from build123d import *

# Parameters (mm, degrees)
F0_R     = 6.35
F1_DEPTH = 19.05


with BuildPart() as f1:
    # F0 (on Front) → F1 (new body)
    with BuildSketch(Plane.XZ):
        with BuildLine():
            ThreePointArc((6.35, -50.8), (4.490128, -46.309872), (0, -44.45))
            ThreePointArc((0, -44.45), (-4.490128, -55.290128), (6.35, -50.8))
        make_face()
        with Locations((-50.8, 0)):
            Circle(F0_R)
        with BuildLine():
            ThreePointArc((6.35, 50.8), (-4.490128, 55.290128), (0, 44.45))
            ThreePointArc((0, 44.45), (4.490128, 46.309872), (6.35, 50.8))
        make_face()
        with BuildLine():
            ThreePointArc((57.15, 0), (50.8, 6.35), (44.45, 0))
            ThreePointArc((44.45, 0), (50.8, -6.35), (57.15, 0))
        make_face()
        with BuildLine():
            ThreePointArc((12.883376, 50.8), (9.109922, 59.909922), (0, 63.683376))
            ThreePointArc((0, 63.683376), (-9.109922, 59.909922), (-12.883376, 50.8))
            ThreePointArc((-12.883376, 50.8), (-21.70632, 21.661631), (-50.8, 12.692425))
            ThreePointArc((-50.8, 12.692425), (-59.7749, 8.9749), (-63.492425, 0))
            ThreePointArc((-63.492425, 0), (-59.7749, -8.9749), (-50.8, -12.692425))
            ThreePointArc((-50.8, -12.692425), (-22.664281, -22.614792), (-12.883376, -50.8))
            ThreePointArc((-12.883376, -50.8), (-9.109922, -59.909922), (0, -63.683376))
            ThreePointArc((0, -63.683376), (9.109922, -59.909922), (12.883376, -50.8))
            ThreePointArc((12.883376, -50.8), (22.285467, -22.332575), (50.8, -13.074334))
            ThreePointArc((50.8, -13.074334), (60.04495, -9.24495), (63.874334, 0))
            ThreePointArc((63.874334, 0), (60.04495, 9.24495), (50.8, 13.074334))
            ThreePointArc((50.8, 13.074334), (21.896637, 21.941776), (12.883376, 50.8))
        make_face()
        with BuildLine():
            ThreePointArc((6.35, -50.8), (-4.490128, -55.290128), (0, -44.45))
            ThreePointArc((0, -44.45), (4.490128, -46.309872), (6.35, -50.8))
        make_face(mode=Mode.SUBTRACT)
        with Locations((-50.8, 0)):
            Circle(F0_R, mode=Mode.SUBTRACT)
        with BuildLine():
            ThreePointArc((0, 12.7), (8.980256, 8.980256), (12.7, 0))
            ThreePointArc((12.7, 0), (8.980256, -8.980256), (0, -12.7))
            ThreePointArc((0, -12.7), (-8.980256, -8.980256), (-12.7, 0))
            ThreePointArc((-12.7, 0), (-8.980256, 8.980256), (0, 12.7))
        make_face(mode=Mode.SUBTRACT)
        with BuildLine():
            ThreePointArc((6.35, 50.8), (4.490128, 46.309872), (0, 44.45))
            ThreePointArc((0, 44.45), (-4.490128, 55.290128), (6.35, 50.8))
        make_face(mode=Mode.SUBTRACT)
        with BuildLine():
            ThreePointArc((57.15, 0), (50.8, -6.35), (44.45, 0))
            ThreePointArc((44.45, 0), (50.8, 6.35), (57.15, 0))
        make_face(mode=Mode.SUBTRACT)
    extrude(amount=F1_DEPTH)


solid = f1.part
Design review of the part built by this model. Coordinates are the model's own, in mm. Round coordinates to 2 decimals unless told otherwise and drop trailing zeros. Write each loop counter-clockwise with the first axis right and the second up, starting at its lowest first coordinate (ties: lowest second). Pieces come first, ordered by that corner, then holes. Notation, with made-up numbers: (61, 6) - (111, 6) arc R3 ccw to (111, 10) - close; hole circle Ø6 at (18.5, 4). An arc over 180 degrees is marked (long way). Return JSON: item names as keys, results as strings. Group by question number.
Item 1: We need section A-A on y = -7.25. Write out the cut boundary in (x, z), and give its area (3 significant figures).
Item 2: We need section B-B on x = 20.5. Write out the cut boundary in (y, z).
Item 3: For probe 1 along Z at (x, y) = (2, -16); probe 2 along Z at (x, y) = (50.8, -10); probe 3 along Z at (x, y) = (-50.8, -4.5), list the stretches that pass through material, from the lowest coordinate up. Write a range as [from, to].
Item 4: The part is to be moulded in two halves that separate along Z. For faces 1 (the face through (-21.396, -9.392, 21.978)), 2 (the face through (-14, -19.05, -4)), say which applies: pulls with the +Z half, pulls with the -Z half, needs draft (parallel to the pull), parting line crosses it, or undercut.
Item 5: Insertion check: P1, Ø11.5, axis at x = 0, z = 50.8, coming from the -Y side; P2, Ø1.5, axis at x = 36.5, y = -4, coming from the +Z side; P3, Ø8, axis at y = -7, z = -44.5, coming from the +X side; P4, Ø10, axis at y = -9, z = 26, coming from the +X side. Each pin has a flat end and moves straight along its axis. Give the tip position at first contact, or say it passes through.
Item 6: We need section C-C on z = 18. Write out the cut boundary in (x, y), and give its area (4 significant figures).
Model answer:
{
 "1": {"outline": "(-63.49, 0) arc R12.69 ccw to (-50.8, -12.69) arc R34.38 cw to (-12.88, -50.8) arc R12.88 ccw to (0, -63.68) arc R12.88 ccw to (12.88, -50.8) arc R33.17 cw to (50.8, -13.07) arc R13.07 ccw to (63.87, 0) arc R13.07 ccw to (50.8, 13.07) arc R32.41 cw to (12.88, 50.8) arc R12.88 ccw to (0, 63.68) arc R12.88 ccw to (-12.88, 50.8) arc R32.41 cw to (-50.8, 12.69) arc R12.69 ccw to start; hole circle Ø12.7 at (-50.8, 0); hole circle Ø25.4 at (0, 0); hole circle Ø12.7 at (0, -50.8); hole circle Ø12.7 at (0, 50.8); hole circle Ø12.7 at (50.8, 0)", "area": "5,410 mm²"},
 "2": {"outline": "(-19.05, -24.26) - (0, -24.26) - (0, 23.42) - (-19.05, 23.42) - close"},
 "3": {"probe 1": "z = [-63.53, -56.83], [-44.77, -12.54], [12.54, 44.77], [56.83, 63.53]", "probe 2": "z = [-13.07, -6.35], [6.35, 13.07]", "probe 3": "z = [-12.69, -6.35], [6.35, 12.69]"},
 "4": {"face 1": "undercut", "face 2": "needs draft"},
 "5": {"P1": "passes through", "P2": "stops at z = 13.78", "P3": "stops at x = 12.94", "P4": "stops at x = 22.88"},
 "6": {"outline": "(-26.05, -19.05) - (26.7, -19.05) - (26.7, 0) - (-26.05, 0) - close", "area": "1,005 mm²"}
}
